```python
from build123d import *

# Parameters (mm, degrees)
SKETCH1_W                     = 241.3
SKETCH1_H                     = 190.5
MAIN_BODY_DEPTH               = 1.5875
SKETCH2_R                     = 2.286
BOLT_HOLES_DEPTH              = 2.5875
SKETCH3_R                     = 2.286
LOCKING_MECHANISM_HOLES_DEPTH = 2.5875
SKETCH4_W                     = 12.7
SKETCH4_H                     = 12.7
LED_HOLES_DEPTH               = 2.5875
SKETCH5_R                     = 1.27
LOGO_MOUNT_HOLES_DEPTH        = 2.5875
SKETCH6_R                     = 5.08
PANEL_MOUNT_LED_HOLE_DEPTH    = 2.5875


with BuildPart() as part:
    # Sketch1 → Main Body (new body)
    with BuildSketch(Plane(origin=(0, 0, 0), x_dir=(0, 0, -1), z_dir=(1, 0, 0))):
        with Locations((120.65, 95.25)):
            Rectangle(SKETCH1_W, SKETCH1_H)
    extrude(amount=MAIN_BODY_DEPTH)

    # Sketch2 → Bolt Holes (cut, through all)
    with BuildSketch(Plane(origin=(1.5875, 0, 0), x_dir=(0, 0, -1), z_dir=(1, 0, 0))):
        with Locations((227.0125, 14.2875)):
            Circle(SKETCH2_R)
        with Locations((227.0125, 176.2125)):
            Circle(SKETCH2_R)
        with Locations((14.2875, 14.2875)):
            Circle(SKETCH2_R)
        with Locations((14.2875, 176.2125)):
            Circle(SKETCH2_R)
    extrude(amount=-BOLT_HOLES_DEPTH, mode=Mode.SUBTRACT)

    # Sketch3 → Locking Mechanism Holes (cut, through all)
    with BuildSketch(Plane(origin=(1.5875, 0, 0), x_dir=(0, 0, -1), z_dir=(1, 0, 0))):
        with Locations((63.246, 181.2925)):
            Circle(SKETCH3_R)
        with Locations((82.55, 181.2925)):
            Circle(SKETCH3_R)
        with Locations((158.75, 181.2925)):
            Circle(SKETCH3_R)
        with Locations((178.054, 181.2925)):
            Circle(SKETCH3_R)
    extrude(amount=-LOCKING_MECHANISM_HOLES_DEPTH, mode=Mode.SUBTRACT)

    # Sketch4 → LED Holes (cut, through all)
    with BuildSketch(Plane(origin=(1.5875, 0, 0), x_dir=(0, 0, -1), z_dir=(1, 0, 0))):
        with Locations((25.4, 95.25)):
            Rectangle(SKETCH4_W, SKETCH4_H)
        with Locations((215.9, 95.25)):
            Rectangle(SKETCH4_W, SKETCH4_H)
    extrude(amount=-LED_HOLES_DEPTH, mode=Mode.SUBTRACT)

    # Sketch5 → Logo Mount Holes (cut, through all)
    with BuildSketch(Plane(origin=(1.5875, 0, 0), x_dir=(0, 0, -1), z_dir=(1, 0, 0))):
        with Locations((120.65, 157.48)):
            Circle(SKETCH5_R)
        with Locations((120.65, 33.02)):
            Circle(SKETCH5_R)
    extrude(amount=-LOGO_MOUNT_HOLES_DEPTH, mode=Mode.SUBTRACT)

    # Sketch6 → Panel Mount LED Hole (cut, through all)
    with BuildSketch(Plane(origin=(1.5875, 0, 0), x_dir=(0, 0, -1), z_dir=(1, 0, 0))):
        with Locations((38.1, 25.4)):
            Circle(SKETCH6_R)
        with Locations((53.34, 25.4)):
            Circle(SKETCH6_R)
        with Locations((68.58, 25.4)):
            Circle(SKETCH6_R)
    extrude(amount=-PANEL_MOUNT_LED_HOLE_DEPTH, mode=Mode.SUBTRACT)


solid = part.part
```
Can you work these out from the model? Positions are in its coordinate system, mm. Coordinates: 2 decimals unless noted, no trailing zeros. Order: outer loops, then holes, each group sorted by start corner. A loop starts at its lowest first (then second) coordinate and runs counter-clockwise, first axis right, second up.
1. I'm going to push a flat-ended pin straight in: pin 1 (4 mm diameter, centred on y = 14.29, z = -14.29, fed in from +X). Where does the tip first touch, or does it pass through?
2. If we section it at B-B (z = -38.1): Please give me the cut outline in (x, y).
3. I need wall thicknesses on line 1 (Y direction, x = 1.05, z = -120.65); line 2 (Y direction, x = 0.6, z = -158.75); line 3 (Y direction, x = 1, z = -211.5). Which ranges of each line are inside material? Lowest first, please.
4. If we section it at A-A (y = 25.4): Please give me the cut outline in (x, z).
5. Thinking about a two-plate mould opening in Y: for faces 1 (the face through (1.588, 97, -119)), 2 (the face through (0.805, 25.623, -63.505)), which applies, +Y half, -Y half, draft (parallel to the pull), parting line (faces both ways), or undercut?
6. If we section it at C-C (x = 0.85): Give the number of separate pieces and of enclosed holes in the cut face, then the cut area to 3 significant figures.
Entries:
1. pin 1: passes through
2. outline: (0, 0) - (1.59, 0) - (1.59, 20.32) - (0, 20.32) - close; (0, 30.48) - (1.59, 30.48) - (1.59, 190.5) - (0, 190.5) - close
3. line 1: y = 0 to 31.75, 34.29 to 156.21, 158.75 to 190.5
3. line 2: y = 0 to 179.01, 183.58 to 190.5
3. line 3: y = 0 to 88.9, 101.6 to 190.5
4. outline: (0, -241.3) - (1.59, -241.3) - (1.59, -73.66) - (0, -73.66) - close; (0, -63.5) - (1.59, -63.5) - (1.59, -58.42) - (0, -58.42) - close; (0, -48.26) - (1.59, -48.26) - (1.59, -43.18) - (0, -43.18) - close; (0, -33.02) - (1.59, -33.02) - (1.59, 0) - (0, 0) - close
5. face 1: draft
5. face 2: undercut
6. separate pieces: 1
6. enclosed holes: 15
6. area: 45,300 mm2
